Could you check a few things on this model? Use its own coordinates, in mm. Face numbers are marked on the shaded views. A direction names the side the tool comes from. Give positions to 0.01 mm unless a question says otherwise; leave off trailing zeros. Write each loop counter-clockwise with the first axis right and the second up, starting at its lowest first coordinate (ties: lowest second). Pieces come first, ordered by that corner, then holes. Notation, with made-up numbers: M 64,82.5 L 117,82.5 A31 cw 117,111.5 Z; hole C -34,16.5 d7. An arc over 180 degrees is marked long. One line per item, written item: value.
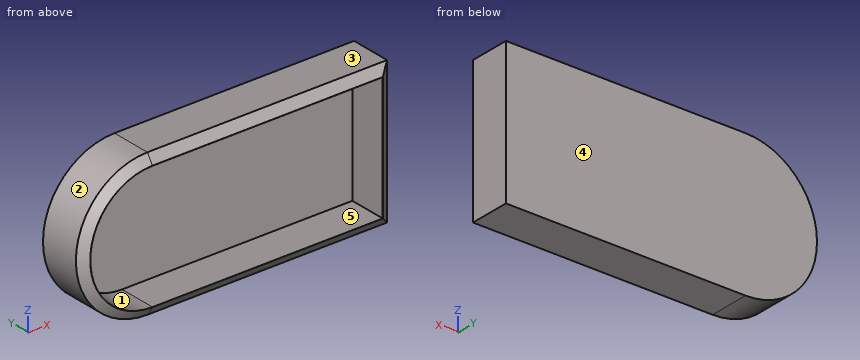
```python
from build123d import *
from OCP.BRepFilletAPI import BRepFilletAPI_MakeChamfer

# Parameters (mm, degrees)
BOSS_EXTRUDE1_DEPTH = 3
BOSS_EXTRUDE3_START = -15
BOSS_EXTRUDE3_DEPTH = 15
CHAMFER2_SIZE       = 2
CHAMFER2_SIZE2      = 2.965121937


with BuildPart() as part:
    # Sketch1 → Boss-Extrude1 (new body)
    with BuildSketch(Plane(origin=(0, 0, 0), x_dir=(1, 0, 0), z_dir=(0, 1, 0))):
        with BuildLine():
            Line((20.272183792, 10.837794599), (-53.767816208, 10.837794599))
            ThreePointArc((-53.767816208, 10.837794599), (-39.625680584, 4.979930223), (-33.767816208, -9.162205401))
            ThreePointArc((-33.767816208, -9.162205401), (-39.625680584, -23.304341024), (-53.767816208, -29.162205401))
            Line((-53.767816208, -29.162205401), (20.272183792, -29.162205401))
            Line((20.272183792, -29.162205401), (20.272183792, 10.837794599))
        make_face()
        with BuildLine():
            ThreePointArc((-33.767816208, -9.162205401), (-39.625680584, 4.979930223), (-53.767816208, 10.837794599))
            Line((-53.767816208, 10.837794599), (-53.767816208, -29.162205401))
            ThreePointArc((-53.767816208, -29.162205401), (-39.625680584, -23.304341024), (-33.767816208, -9.162205401))
        make_face()
        with BuildLine():
            Line((-53.767816208, -29.162205401), (-53.767816208, 10.837794599))
            ThreePointArc((-53.767816208, 10.837794599), (-73.767816208, -9.162205401), (-53.767816208, -29.162205401))
        make_face()
        with BuildLine():
            ThreePointArc((-33.767816208, -9.162205401), (-39.625680584, 4.979930223), (-53.767816208, 10.837794599))
            Line((-53.767816208, 10.837794599), (-53.767816208, -29.162205401))
            ThreePointArc((-53.767816208, -29.162205401), (-39.625680584, -23.304341024), (-33.767816208, -9.162205401))
        make_face()
        with BuildLine():
            Line((-53.767816208, -29.162205401), (-53.767816208, 10.837794599))
            ThreePointArc((-53.767816208, 10.837794599), (-73.767816208, -9.162205401), (-53.767816208, -29.162205401))
        make_face()
    extrude(amount=BOSS_EXTRUDE1_DEPTH)

    # Sketch2 → Boss-Extrude3 (add)
    with BuildSketch(Plane(origin=(0, 3, 0), x_dir=(1, 0, 0), z_dir=(0, 1, 0)).offset(BOSS_EXTRUDE3_START)):
        with BuildLine():
            ThreePointArc((-53.767816208, -29.162205401), (-73.767816208, -9.162205401), (-53.767816208, 10.837794599))
            Line((-53.767816208, 10.837794599), (-53.767816208, 13.837794599))
            ThreePointArc((-53.767816208, 13.837794599), (-76.767816208, -9.162205401), (-53.767816208, -32.162205401))
            Line((-53.767816208, -32.162205401), (-53.767816208, -29.162205401))
        make_face()
        with BuildLine():
            Line((-53.767816208, 13.837794599), (-53.767816208, 10.837794599))
            Line((-53.767816208, 10.837794599), (-42.409999516, 10.837794599))
            ThreePointArc((-42.409999516, 10.837794599), (-47.894146145, 13.075150557), (-53.767816208, 13.837794599))
        make_face()
        with BuildLine():
            Line((-42.409999516, -29.162205401), (-53.767816208, -29.162205401))
            Line((-53.767816208, -29.162205401), (-53.767816208, -32.162205401))
            ThreePointArc((-53.767816208, -32.162205401), (-47.894146145, -31.399561359), (-42.409999516, -29.162205401))
        make_face()
        with BuildLine():
            Line((23.272183792, 13.837794599), (-53.767816208, 13.837794599))
            ThreePointArc((-53.767816208, 13.837794599), (-47.894146145, 13.075150557), (-42.409999516, 10.837794599))
            Line((-42.409999516, 10.837794599), (20.272183792, 10.837794599))
            Line((20.272183792, 10.837794599), (20.272183792, -29.162205401))
            Line((20.272183792, -29.162205401), (-42.409999516, -29.162205401))
            ThreePointArc((-42.409999516, -29.162205401), (-47.894146145, -31.399561359), (-53.767816208, -32.162205401))
            Line((-53.767816208, -32.162205401), (23.272183792, -32.162205401))
            Line((23.272183792, -32.162205401), (23.272183792, 13.837794599))
        make_face()
    extrude(amount=BOSS_EXTRUDE3_DEPTH)

    # Chamfer2: one chamfer whose edges measure the first distance from different faces: ONE call of the kernel's chamfer builder (chamfer() names one face for all edges)
    chamfer2_edges_1 = [part.edges().sort_by_distance(p)[0] for p in [
        (-76.767816208, -12, 9.162205401),
    ]]
    chamfer2_side_1 = [part.faces().sort_by_distance(p)[0] for p in [
        (-76.767816208, -4.5, 9.162205401),
    ]]
    chamfer2_edges_2 = [part.edges().sort_by_distance(p)[0] for p in [
        (-15.247816208, -12, -13.837794599),
    ]]
    chamfer2_side_2 = [part.faces().sort_by_distance(p)[0] for p in [
        (-15.247816208, -4.5, -13.837794599),
    ]]
    chamfer2_edges_3 = [part.edges().sort_by_distance(p)[0] for p in [
        (23.272183792, -12, 9.162205401),
    ]]
    chamfer2_side_3 = [part.faces().sort_by_distance(p)[0] for p in [
        (23.272183792, -4.5, 9.162205401),
    ]]
    chamfer2_edges_4 = [part.edges().sort_by_distance(p)[0] for p in [
        (-15.247816208, -12, 32.162205401),
    ]]
    chamfer2_side_4 = [part.faces().sort_by_distance(p)[0] for p in [
        (-15.247816208, -4.5, 32.162205401),
    ]]
    chamfer2 = BRepFilletAPI_MakeChamfer(part.part.solid().wrapped)
    for e in chamfer2_edges_1:
        chamfer2.Add(CHAMFER2_SIZE, CHAMFER2_SIZE2, e.wrapped, chamfer2_side_1[0].wrapped)  # the first distance lies on this face
    for e in chamfer2_edges_2:
        chamfer2.Add(CHAMFER2_SIZE, CHAMFER2_SIZE2, e.wrapped, chamfer2_side_2[0].wrapped)  # the first distance lies on this face
    for e in chamfer2_edges_3:
        chamfer2.Add(CHAMFER2_SIZE, CHAMFER2_SIZE2, e.wrapped, chamfer2_side_3[0].wrapped)  # the first distance lies on this face
    for e in chamfer2_edges_4:
        chamfer2.Add(CHAMFER2_SIZE, CHAMFER2_SIZE2, e.wrapped, chamfer2_side_4[0].wrapped)  # the first distance lies on this face
    add(Compound.cast(chamfer2.Shape()), mode=Mode.REPLACE)


solid = part.part
```
1) If we section it at C-C, the plane y = 2: Write out the boundary of the cut face in (x, z), then the cut area to 3 significant figures.
Outcome:
outline: M -53.77,-13.84 L 23.27,-13.84 L 23.27,32.16 L -53.77,32.16 A23 ccw Z
area: 4,370 mm^2
2) I'm going to push flat-ended pins straight in: pin 1 (4 mm diameter, centred on y = -1, z = 6.5, fed in from -X); pin 2 (2 mm diameter, centred on x = -53, z = 25.5, fed in from -Y); pin 3 (3 mm diameter, centred on y = -7, z = 5.5, fed in from -X). Where does each tip first touch, or does it pass through?
Outcome:
pin 1: stops at x = -76.76
pin 2: stops at y = 0
pin 3: stops at x = -76.67
3) If we section it at A-A, the plane y = -4.75: Write out the boundary of the cut face in (x, z), then the cut area to 3 significant figures.
Outcome:
outline: M -53.77,-13.84 L 23.27,-13.84 L 23.27,32.16 L -53.77,32.16 A23 ccw Z; hole M -53.77,-10.84 L 20.27,-10.84 L 20.27,29.16 L -53.77,29.16 A20 ccw Z
area: 785 mm^2
4) Please list where these lines run through material, in increasing order: L1, parallel to Z at x = -40, y = -2; L2, parallel to Y at x = -36, z = -9; L3, parallel to X at y = -5, z = 6. Write a range as from..to.
Outcome:
L1: z = -13.84..-10.84, 29.16..32.16
L2: y = 0..3
L3: x = -76.55..-73.52, 20.27..23.27
5) On a 3-axis mill with a long thin cutter (end or side, diameter ignored), from which of +Z, -Z, +X, -X, +Y, -Y can I reach the whole of each face in a straight line? I mean the marked faces 4 and 5. Say none if no direction works.
Outcome:
face 4: +Z, -Z, +X, -X, +Y
face 5: -Y
6) We'd pull the mould along X, two halves only. Please class the marked faces 1, 2 and 3: pulls with the +X half, pulls with the -X half, needs draft (parallel to the pull), parting line crosses it, or undercut.
Outcome:
face 1: undercut
face 2: pulls with the -X half
face 3: needs draft
